Build history of the part. All positions in model axes, mm. Give positions to 0.01 mm unless a question says otherwise; leave off trailing zeros. Order: outer loops, then holes, each group sorted by start corner. A loop starts at its lowest first (then second) coordinate and runs counter-clockwise, first axis right, second up. Notation, with made-up numbers: (41.5, 4.25) -> (53.5, 4.25) arc R34 cw to (53.5, 37.25) -> close; hole circle Ø8 at (71, 60.25). An arc over 180 degrees is marked (long way). Use a Markdown table: item, result. Add a question column.
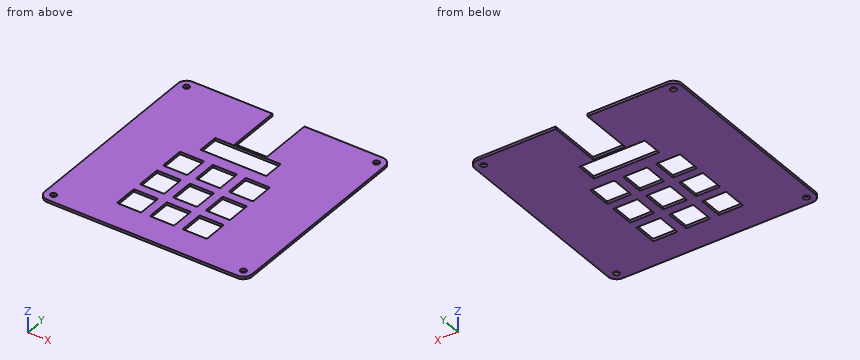
Autodesk Inventor part; units mm, degrees
ref_plane "YZ Plane" through (0, 0, 0) normal (1, 0, 0) x (0, 1, 0)
ref_plane "XZ Plane" through (0, 0, 0) normal (0, 1, 0) x (-1, 0, 0)
ref_plane "XY Plane" through (0, 0, 0) normal (0, 0, 1) x (1, 0, 0)
sketch "Sketch1" plane through (0, 0, 0) normal (0, 0, 1) x (1, 0, 0)
  point P0 (0, 0)
sketch "0" plane through (0, 0, 0) normal (0, 0, 1) x (1, 0, 0)
  line L0 (3.025, -2.525) -> (16.025, -2.525)
  line L1 (3.025, -16.525) -> (16.025, -16.525)
  line L2 (2.525, -3.025) -> (2.525, -16.025)
  line L3 (16.525, -3.025) -> (16.525, -16.025)
  arc A0 (3.025, -2.525) -> (2.525, -3.025) centre (3.025, -3.025) ccw
  arc A1 (16.525, -3.025) -> (16.025, -2.525) centre (16.025, -3.025) ccw
  arc A2 (2.525, -16.025) -> (3.025, -16.525) centre (3.025, -16.025) ccw
  arc A3 (16.025, -16.525) -> (16.525, -16.025) centre (16.025, -16.025) ccw
  line L4 (22.075, -2.525) -> (35.075, -2.525)
  line L5 (22.075, -16.525) -> (35.075, -16.525)
  line L6 (21.575, -3.025) -> (21.575, -16.025)
  line L7 (35.575, -3.025) -> (35.575, -16.025)
  arc A4 (22.075, -2.525) -> (21.575, -3.025) centre (22.075, -3.025) ccw
  arc A5 (35.575, -3.025) -> (35.075, -2.525) centre (35.075, -3.025) ccw
  arc A6 (21.575, -16.025) -> (22.075, -16.525) centre (22.075, -16.025) ccw
  arc A7 (35.075, -16.525) -> (35.575, -16.025) centre (35.075, -16.025) ccw
  line L8 (41.125, -2.525) -> (54.125, -2.525)
  line L9 (41.125, -16.525) -> (54.125, -16.525)
  line L10 (40.625, -3.025) -> (40.625, -16.025)
  line L11 (54.625, -3.025) -> (54.625, -16.025)
  arc A8 (41.125, -2.525) -> (40.625, -3.025) centre (41.125, -3.025) ccw
  arc A9 (54.625, -3.025) -> (54.125, -2.525) centre (54.125, -3.025) ccw
  arc A10 (40.625, -16.025) -> (41.125, -16.525) centre (41.125, -16.025) ccw
  arc A11 (54.125, -16.525) -> (54.625, -16.025) centre (54.125, -16.025) ccw
  line L12 (3.025, -21.575) -> (16.025, -21.575)
  line L13 (3.025, -35.575) -> (16.025, -35.575)
  line L14 (2.525, -22.075) -> (2.525, -35.075)
  line L15 (16.525, -22.075) -> (16.525, -35.075)
  arc A12 (3.025, -21.575) -> (2.525, -22.075) centre (3.025, -22.075) ccw
  arc A13 (16.525, -22.075) -> (16.025, -21.575) centre (16.025, -22.075) ccw
  arc A14 (2.525, -35.075) -> (3.025, -35.575) centre (3.025, -35.075) ccw
  arc A15 (16.025, -35.575) -> (16.525, -35.075) centre (16.025, -35.075) ccw
  line L16 (22.075, -21.575) -> (35.075, -21.575)
  line L17 (22.075, -35.575) -> (35.075, -35.575)
  line L18 (21.575, -22.075) -> (21.575, -35.075)
  line L19 (35.575, -22.075) -> (35.575, -35.075)
  arc A16 (22.075, -21.575) -> (21.575, -22.075) centre (22.075, -22.075) ccw
  arc A17 (35.575, -22.075) -> (35.075, -21.575) centre (35.075, -22.075) ccw
  arc A18 (21.575, -35.075) -> (22.075, -35.575) centre (22.075, -35.075) ccw
  arc A19 (35.075, -35.575) -> (35.575, -35.075) centre (35.075, -35.075) ccw
  line L20 (41.125, -21.575) -> (54.125, -21.575)
  line L21 (41.125, -35.575) -> (54.125, -35.575)
  line L22 (40.625, -22.075) -> (40.625, -35.075)
  line L23 (54.625, -22.075) -> (54.625, -35.075)
  arc A20 (41.125, -21.575) -> (40.625, -22.075) centre (41.125, -22.075) ccw
  arc A21 (54.625, -22.075) -> (54.125, -21.575) centre (54.125, -22.075) ccw
  arc A22 (40.625, -35.075) -> (41.125, -35.575) centre (41.125, -35.075) ccw
  arc A23 (54.125, -35.575) -> (54.625, -35.075) centre (54.125, -35.075) ccw
  line L24 (3.025, -40.625) -> (16.025, -40.625)
  line L25 (3.025, -54.625) -> (16.025, -54.625)
  line L26 (2.525, -41.125) -> (2.525, -54.125)
  line L27 (16.525, -41.125) -> (16.525, -54.125)
  arc A24 (3.025, -40.625) -> (2.525, -41.125) centre (3.025, -41.125) ccw
  arc A25 (16.525, -41.125) -> (16.025, -40.625) centre (16.025, -41.125) ccw
  arc A26 (2.525, -54.125) -> (3.025, -54.625) centre (3.025, -54.125) ccw
  arc A27 (16.025, -54.625) -> (16.525, -54.125) centre (16.025, -54.125) ccw
  line L28 (22.075, -40.625) -> (35.075, -40.625)
  line L29 (22.075, -54.625) -> (35.075, -54.625)
  line L30 (21.575, -41.125) -> (21.575, -54.125)
  line L31 (35.575, -41.125) -> (35.575, -54.125)
  arc A28 (22.075, -40.625) -> (21.575, -41.125) centre (22.075, -41.125) ccw
  arc A29 (35.575, -41.125) -> (35.075, -40.625) centre (35.075, -41.125) ccw
  arc A30 (21.575, -54.125) -> (22.075, -54.625) centre (22.075, -54.125) ccw
  arc A31 (35.075, -54.625) -> (35.575, -54.125) centre (35.075, -54.125) ccw
  line L32 (41.125, -40.625) -> (54.125, -40.625)
  line L33 (41.125, -54.625) -> (54.125, -54.625)
  line L34 (40.625, -41.125) -> (40.625, -54.125)
  line L35 (54.625, -41.125) -> (54.625, -54.125)
  arc A32 (41.125, -40.625) -> (40.625, -41.125) centre (41.125, -41.125) ccw
  arc A33 (54.625, -41.125) -> (54.125, -40.625) centre (54.125, -41.125) ccw
  arc A34 (40.625, -54.125) -> (41.125, -54.625) centre (41.125, -54.125) ccw
  arc A35 (54.125, -54.625) -> (54.625, -54.125) centre (54.125, -54.125) ccw
  line L36 (-30.946, 48.585) -> (89.054, 48.585)
  line L37 (89.054, 48.585) -> (89.054, -71.415)
  line L38 (89.054, -71.415) -> (-30.946, -71.415)
  line L39 (-30.946, -71.415) -> (-30.946, 48.585)
  line L40 (20.309, 48.585) -> (38.809, 48.585)
  line L41 (38.809, 48.585) -> (38.809, 17.585)
  line L42 (38.809, 17.585) -> (20.309, 17.585)
  line L43 (20.309, 17.585) -> (20.309, 48.585)
  circle A36 centre (-25.946, 43.585) radius 1.7
  circle A37 centre (84.054, 43.585) radius 1.7
  circle A38 centre (84.054, -66.415) radius 1.7
  circle A39 centre (-25.946, -66.415) radius 1.7
  line L44 (9.675, 16.395) -> (47.675, 16.395)
  line L45 (47.675, 16.395) -> (47.675, 4.395)
  line L46 (47.675, 4.395) -> (9.675, 4.395)
  line L47 (9.675, 4.395) -> (9.675, 16.395)
  point P0 (9.525, -54.625)
  dimension "d0" = 120
  dimension "d1" = 120
  dimension "d2" = 33.471
  dimension "d3" = 16.79
  dimension "d4" = 18.5
  dimension "d5" = 31
  dimension "d6" = 51.255
  dimension "d7" = 3.4
  dimension "d8" = 3.4
  dimension "d9" = 3.4
  dimension "d10" = 3.4
  dimension "d11" = 5
  dimension "d12" = 5
  dimension "d13" = 5
  dimension "d14" = 5
  dimension "d15" = 5
  dimension "d16" = 5
  dimension "d17" = 5
  dimension "d18" = 5
  dimension "d19" = 38
  dimension "d20" = 12
  dimension "d21" = 40.621
  dimension "d22" = 32.19
extrude "Extrusion1" add sketch "0" along normal blind 1.5 contours L36 L43 L42 L41 L37 L38 L39
fillet "Fillet1" radius 5 4 edges at (-30.946, -71.415, 0.75) (89.054, -71.415, 0.75) (89.054, 48.585, 0.75) (-30.946, 48.585, 0.75)
properties part number "Top_Case_New"
(1) Band-saw the part on B-B on x = 27. Give the cut face in (y, z) (3 decimals), plus the area to 3 significant figures.
(2) Band-saw the part on C-C on y = -27. Give the cut face in (x, z) (3 decimals).
(3) Band-saw the part on A-A on y = 22. Give the cut face in (x, z).
(4) Band-saw the part on D-D on z = 0.75. State how many separate pieces and enclosed holes the cut face has, plus the area to 3 significant figures.
(5) Wall check: probe 1 along X at (y, z) = (-32, 0.4) (3 decimals); probe 2 along Y at (x, z) = (26, 0.9) (3 decimals); probe 3 along Y at (x, z) = (46, 0.2) (3 decimals). Give the ranges that are in metal, low to high.
Response:
| question | item | result |
|---|---|---|
| 1 | outline | (-71.415, 0) -> (-54.625, 0) -> (-54.625, 1.5) -> (-71.415, 1.5) -> close; (-40.625, 0) -> (-35.575, 0) -> (-35.575, 1.5) -> (-40.625, 1.5) -> close; (-21.575, 0) -> (-16.525, 0) -> (-16.525, 1.5) -> (-21.575, 1.5) -> close; (-2.525, 0) -> (4.395, 0) -> (4.395, 1.5) -> (-2.525, 1.5) -> close; (16.395, 0) -> (17.585, 0) -> (17.585, 1.5) -> (16.395, 1.5) -> close |
| 1 | area | 52.5 mm² |
| 2 | outline | (-30.946, 0) -> (2.525, 0) -> (2.525, 1.5) -> (-30.946, 1.5) -> close; (16.525, 0) -> (21.575, 0) -> (21.575, 1.5) -> (16.525, 1.5) -> close; (35.575, 0) -> (40.625, 0) -> (40.625, 1.5) -> (35.575, 1.5) -> close; (54.625, 0) -> (89.054, 0) -> (89.054, 1.5) -> (54.625, 1.5) -> close |
| 3 | outline | (-30.95, 0) -> (20.31, 0) -> (20.31, 1.5) -> (-30.95, 1.5) -> close; (38.81, 0) -> (89.05, 0) -> (89.05, 1.5) -> (38.81, 1.5) -> close |
| 4 | separate pieces | 1 |
| 4 | enclosed holes | 14 |
| 4 | area | 11,600 mm² |
| 5 | probe 1 | x = -30.946 to 2.525, 16.525 to 21.575, 35.575 to 40.625, 54.625 to 89.054 |
| 5 | probe 2 | y = -71.415 to -54.625, -40.625 to -35.575, -21.575 to -16.525, -2.525 to 4.395, 16.395 to 17.585 |
| 5 | probe 3 | y = -71.415 to -54.625, -40.625 to -35.575, -21.575 to -16.525, -2.525 to 4.395, 16.395 to 48.585 |
